```python
from build123d import *

# Parameters (mm, degrees)
SKETCH1_W           = 152.4
SKETCH1_H           = 76.2
SKETCH1_R           = 2.54
SKETCH1_R_2         = 2.38125
SKETCH1_R_3         = 14.2875
BOSS_EXTRUDE1_DEPTH = 6.35
FILLET1_R           = 6.35
SKETCH2_R           = 15.875
CUT_EXTRUDE1_DEPTH  = 1.5875


with BuildPart() as part:
    # Sketch1 → Boss-Extrude1 (new body)
    with BuildSketch(Plane.XY):
        Rectangle(SKETCH1_W, SKETCH1_H)
        with Locations((44.45, 28.575)):
            Circle(SKETCH1_R, mode=Mode.SUBTRACT)
        with Locations((44.45, -28.022317844)):
            Circle(SKETCH1_R, mode=Mode.SUBTRACT)
        with Locations((63.5, 25.4)):
            Circle(SKETCH1_R_2, mode=Mode.SUBTRACT)
        with Locations((63.5, 0)):
            Circle(SKETCH1_R_2, mode=Mode.SUBTRACT)
        with Locations((63.5, -25.4)):
            Circle(SKETCH1_R_2, mode=Mode.SUBTRACT)
        with Locations((-4.550000044, 0.284999938)):
            Circle(SKETCH1_R_3, mode=Mode.SUBTRACT)
        with Locations((-52.950000018, 0.284999938)):
            Circle(SKETCH1_R, mode=Mode.SUBTRACT)
    extrude(amount=BOSS_EXTRUDE1_DEPTH)

    # Fillet1
    fillet1_edges = [part.edges().sort_by_distance(p)[0] for p in [
        (76.2, -38.1, 3.175),
        (-76.2, -38.1, 3.175),
        (-76.2, 38.1, 3.175),
        (76.2, 38.1, 3.175),
    ]]
    fillet(fillet1_edges, radius=FILLET1_R)

    # Sketch2 → Cut-Extrude1 (cut)
    with BuildSketch(Plane.XY.offset(6.35)):
        with Locations((-4.550000044, 0.284999938)):
            Circle(SKETCH2_R)
    extrude(amount=-CUT_EXTRUDE1_DEPTH, mode=Mode.SUBTRACT)


solid = part.part
```
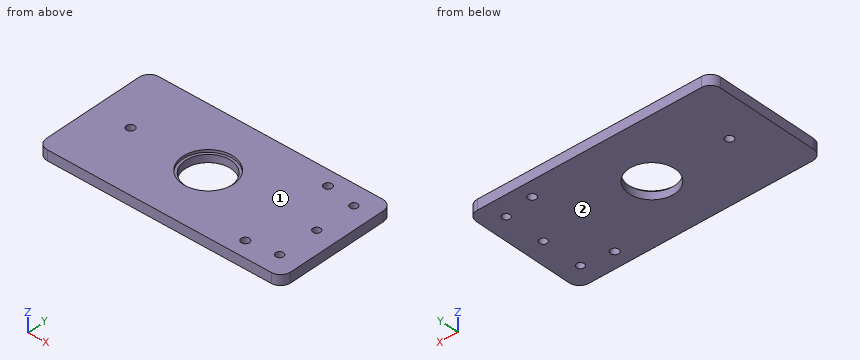
Can you work these out from the model? Positions are in its coordinate system, mm. Face numbers are marked on the shaded views. Give positions to 0.01 mm unless a question says otherwise; leave off trailing zeros. Loops run counter-clockwise (first coordinate to the right, second up) from the corner with the lowest first, then second, coordinate; pieces in that order, holes last. Notation, with made-up numbers: M -23.75,-0.5 L -4.75,-0.5 A28 cw -4.75,35.5 Z; hole C 45.5,7 d5. An arc over 180 degrees is marked long. One line per item, written item: value.
(1) Suppose I cut it at A-A on x = -52.95. List the corners of the cut face in (y, z) for me (3 decimals).
Returned:
outline: M -38.1,0 L -2.255,0 L -2.255,6.35 L -38.1,6.35 Z; M 2.825,0 L 38.1,0 L 38.1,6.35 L 2.825,6.35 Z
(2) Will these pins go through, and if not, where does the flat tip stop? pin 1 (4.5 mm diameter, centred on x = 63.5, y = 25.4, fed in from +Z); pin 2 (1 mm diameter, centred on x = 17.5, y = 18, fed in from -Z).
Returned:
pin 1: through
pin 2: z = 0
(3) Suppose I cut it at D-D on x = 63.5. List the corners of the cut face in (y, z) for me.
Returned:
outline: M -38.1,0 L -27.78,0 L -27.78,6.35 L -38.1,6.35 Z; M -23.02,0 L -2.38,0 L -2.38,6.35 L -23.02,6.35 Z; M 2.38,0 L 23.02,0 L 23.02,6.35 L 2.38,6.35 Z; M 27.78,0 L 38.1,0 L 38.1,6.35 L 27.78,6.35 Z
(4) We'd pull the mould along Z, two halves only. Please class the marked faces 1 and 2: released by +Z, released by -Z, zero draft, split by the parting line, or undercut.
Returned:
face 1: released by +Z
face 2: released by -Z
(5) Suppose I cut it at B-B on x = 44.45. List the corners of the cut face in (y, z) for me (3 decimals), plus the area to 3 significant figures.
Returned:
outline: M -38.1,0 L -30.562,0 L -30.562,6.35 L -38.1,6.35 Z; M -25.482,0 L 26.035,0 L 26.035,6.35 L -25.482,6.35 Z; M 31.115,0 L 38.1,0 L 38.1,6.35 L 31.115,6.35 Z
area: 419 mm^2
(6) I need wall thicknesses on line 1 (Y direction, x = 63.5, z = 2); line 2 (Y direction, x = 44.45, z = 5) (3 decimals); line 3 (Y direction, x = -4.55, z = 5.25). Which ranges of each line are inside material? Lowest first, please.
Returned:
line 1: -38.1 to -27.78, -23.02 to -2.38, 2.38 to 23.02, 27.78 to 38.1
line 2: -38.1 to -30.562, -25.482 to 26.035, 31.115 to 38.1
line 3: -38.1 to -15.59, 16.16 to 38.1
(7) Suppose I cut it at C-C on z = 3. Count the separate pieces of the cut face and the enclosed holes in it, plus the area to 3 significant figures.
Returned:
separate pieces: 1
enclosed holes: 7
area: 10,800 mm^2
